Geometry check sheet. Reference: the model listing, model coordinates, mm. Round coordinates to 2 decimals unless told otherwise and drop trailing zeros. Order: outer loops, then holes, each group sorted by start corner. A loop starts at its lowest first (then second) coordinate and runs counter-clockwise, first axis right, second up.
```python
from build123d import *

# Parameters (mm, degrees)
SKETCH1_R           = 2.54
SKETCH1_R_2         = 2.0193
SKETCH1_R_3         = 14.3002
BOSS_EXTRUDE1_DEPTH = 3.175


with BuildPart() as part:
    # Sketch1 → Boss-Extrude1 (new body)
    with BuildSketch(Plane.XY):
        Polygon((-59.693768546, 4.271271353), (-59.693768546, -46.528728647), (128.614138554, -46.528728647), (292.911431822, 117.768564621), (256.990407338, 153.689589105), (107.572089586, 4.271271353), align=None)
        with Locations((24.040159799, -14.512116048)):
            Circle(SKETCH1_R, mode=Mode.SUBTRACT)
        with Locations((74.840159799, -14.512116048)):
            Circle(SKETCH1_R, mode=Mode.SUBTRACT)
        with Locations((87.540159799, -14.512116048)):
            Circle(SKETCH1_R, mode=Mode.SUBTRACT)
        with Locations((100.240159799, -14.512116048)):
            Circle(SKETCH1_R, mode=Mode.SUBTRACT)
        with Locations((100.240159799, -27.212116048)):
            Circle(SKETCH1_R, mode=Mode.SUBTRACT)
        with Locations((87.540159799, -27.212116048)):
            Circle(SKETCH1_R, mode=Mode.SUBTRACT)
        with Locations((74.840159799, -27.212116048)):
            Circle(SKETCH1_R, mode=Mode.SUBTRACT)
        with Locations((24.040159799, -27.212116048)):
            Circle(SKETCH1_R, mode=Mode.SUBTRACT)
        with Locations((11.340159799, -27.212116048)):
            Circle(SKETCH1_R, mode=Mode.SUBTRACT)
        with Locations((11.340159799, -14.512116048)):
            Circle(SKETCH1_R, mode=Mode.SUBTRACT)
        with Locations((11.158871814, -1.812116048)):
            Circle(SKETCH1_R, mode=Mode.SUBTRACT)
        with Locations((24.040159799, -1.812116048)):
            Circle(SKETCH1_R, mode=Mode.SUBTRACT)
        with Locations((36.558871814, -1.812116048)):
            Circle(SKETCH1_R, mode=Mode.SUBTRACT)
        with Locations((49.258871814, -1.812116048)):
            Circle(SKETCH1_R, mode=Mode.SUBTRACT)
        with Locations((61.958871814, -1.812116048)):
            Circle(SKETCH1_R, mode=Mode.SUBTRACT)
        with Locations((87.540159799, -1.812116048)):
            Circle(SKETCH1_R, mode=Mode.SUBTRACT)
        with Locations((100.058871814, -1.812116048)):
            Circle(SKETCH1_R, mode=Mode.SUBTRACT)
        with Locations((112.758871814, -1.812116048)):
            Circle(SKETCH1_R, mode=Mode.SUBTRACT)
        with Locations((112.758871814, -14.512116048)):
            Circle(SKETCH1_R, mode=Mode.SUBTRACT)
        with Locations((112.758871814, -27.212116048)):
            Circle(SKETCH1_R, mode=Mode.SUBTRACT)
        with Locations((112.758871814, -39.912116048)):
            Circle(SKETCH1_R, mode=Mode.SUBTRACT)
        with Locations((100.058871814, -39.912116048)):
            Circle(SKETCH1_R, mode=Mode.SUBTRACT)
        with Locations((87.540159799, -39.912116048)):
            Circle(SKETCH1_R, mode=Mode.SUBTRACT)
        with Locations((61.958871814, -39.912116048)):
            Circle(SKETCH1_R, mode=Mode.SUBTRACT)
        with Locations((49.258871814, -39.912116048)):
            Circle(SKETCH1_R, mode=Mode.SUBTRACT)
        with Locations((24.040159799, -39.912116048)):
            Circle(SKETCH1_R, mode=Mode.SUBTRACT)
        with Locations((11.158871814, -39.912116048)):
            Circle(SKETCH1_R, mode=Mode.SUBTRACT)
        with Locations((-1.541128186, -39.912116048)):
            Circle(SKETCH1_R, mode=Mode.SUBTRACT)
        with Locations((-1.541128186, -27.212116048)):
            Circle(SKETCH1_R, mode=Mode.SUBTRACT)
        with Locations((-1.541128186, -14.512116048)):
            Circle(SKETCH1_R, mode=Mode.SUBTRACT)
        with Locations((-1.541128186, -1.812116048)):
            Circle(SKETCH1_R, mode=Mode.SUBTRACT)
        with Locations((73.378301019, -3.178216405)):
            Circle(SKETCH1_R_2, mode=Mode.SUBTRACT)
        with Locations((80.817788776, -21.138728647)):
            Circle(SKETCH1_R_2, mode=Mode.SUBTRACT)
        with Locations((73.378301019, -39.099240889)):
            Circle(SKETCH1_R_2, mode=Mode.SUBTRACT)
        with Locations((37.457276534, -39.099240889)):
            Circle(SKETCH1_R_2, mode=Mode.SUBTRACT)
        with Locations((30.017788776, -21.138728647)):
            Circle(SKETCH1_R_2, mode=Mode.SUBTRACT)
        with Locations((55.2538213, -21.128728647)):
            Circle(SKETCH1_R_3, mode=Mode.SUBTRACT)
        with Locations((-32.8841787, -21.128728647)):
            Circle(SKETCH1_R_3, mode=Mode.SUBTRACT)
        with Locations((257.120708411, 117.898865694)):
            Circle(SKETCH1_R_3, mode=Mode.SUBTRACT)
        with Locations((141.58879302, -19.431025607)):
            Circle(SKETCH1_R, mode=Mode.SUBTRACT)
        with Locations((150.569049141, -10.450769486)):
            Circle(SKETCH1_R, mode=Mode.SUBTRACT)
        with Locations((159.549305262, -1.470513365)):
            Circle(SKETCH1_R, mode=Mode.SUBTRACT)
        with Locations((168.529561384, 7.509742756)):
            Circle(SKETCH1_R, mode=Mode.SUBTRACT)
        with Locations((177.509817505, 16.489998877)):
            Circle(SKETCH1_R, mode=Mode.SUBTRACT)
        with Locations((186.490073626, 25.470254998)):
            Circle(SKETCH1_R, mode=Mode.SUBTRACT)
        with Locations((195.470329747, 34.45051112)):
            Circle(SKETCH1_R, mode=Mode.SUBTRACT)
        with Locations((204.450585868, 43.430767241)):
            Circle(SKETCH1_R, mode=Mode.SUBTRACT)
        with Locations((213.430841989, 52.411023362)):
            Circle(SKETCH1_R, mode=Mode.SUBTRACT)
        with Locations((222.41109811, 61.391279483)):
            Circle(SKETCH1_R, mode=Mode.SUBTRACT)
        with Locations((231.391354231, 70.371535604)):
            Circle(SKETCH1_R, mode=Mode.SUBTRACT)
        with Locations((240.371610352, 79.351791725)):
            Circle(SKETCH1_R, mode=Mode.SUBTRACT)
    extrude(amount=BOSS_EXTRUDE1_DEPTH)


solid = part.part
```
(1) Material ranges on line 1 (Y direction, x = 103, z = 2.6); line 2 (Y direction, x = 117, z = 0.6); line 3 (Y direction, x = 170, z = 0.1), recorded low to high.
Returned:
line 1: y = -46.53 to 4.27
line 2: y = -46.53 to 13.7
line 3: y = -5.14 to 5.44, 9.58 to 66.7
(2) Depth check by flat-ended pin: P1, Ø1.6, axis at x = -6, z = 1, coming from the +Y side. Enter the tip coordinate at first touch or a pass-through.
Returned:
P1: stops at y = 4.27
(3) Sectioned sample at B-B, the plane x = 253. Record the cut outline in (y, z) (1 decimal).
Returned:
outline: (77.9, 0) - (104.2, 0) - (104.2, 3.2) - (77.9, 3.2) - close; (131.6, 0) - (149.7, 0) - (149.7, 3.2) - (131.6, 3.2) - close
(4) Sectioned sample at A-A, the plane y = 108. Record the cut outline in (x, z) (3 decimals).
Returned:
outline: (211.301, 0) - (246.8, 0) - (246.8, 3.175) - (211.301, 3.175) - close; (267.441, 0) - (283.143, 0) - (283.143, 3.175) - (267.441, 3.175) - close
(5) Sectioned sample at C-C, the plane z = 0.8. Give the number of separate pieces and of enclosed holes in the cut face, and give its area (3 significant figures).
Returned:
separate pieces: 1
enclosed holes: 51
area: 17,400 mm2
(6) Draft check along X on faces 1 (the flat face through (183.3, 80, 1.6)), 2 (the cylindrical face through (270.33, 112.42, 1.57)), 3 (the flat face through (209.613, 34.47, 1.565)). Enter one of: released by +X, released by -X, zero draft, split by the parting line, or undercut.
Returned:
face 1: released by -X
face 2: undercut
face 3: released by +X
